Design review of the part built by this model. Coordinates are the model's own, in mm. Coordinates: 2 decimals unless noted, no trailing zeros. Loops run counter-clockwise (first coordinate to the right, second up) from the corner with the lowest first, then second, coordinate; pieces in that order, holes last. Notation, with made-up numbers: M -6,20.25 L 18,20.25 A31 ccw 18,48.25 Z; hole C 88,40 d9. An arc over 180 degrees is marked long. Answer as a JSON object with one key per item and string values. Group by question number.
1. To check wall thickness, follow probe 1 along Y at (x, z) = (1.25, 1); probe 2 along Y at (x, z) = (0.25, 0.35); probe 3 along X at (y, z) = (1, 0.5). State the ranges of each line that lie inside material, in increasing order.
2. Insertion check: pin 1 (1 mm diameter, centred on x = 1.5, z = 1.5, fed in from -Y); pin 2 (3 mm diameter, centred on x = 0, y = 0, fed in from +Z). Each pin has a flat end and moves straight along its axis. Give the tip position at first contact, or say it passes through.
3. Consider section B-B (z = 2.7). State the section outline as (x, y) points, then the cut area to 3 significant figures.
4. Consider section A-A (z = 1.35). State the section outline as (x, y) points.
5. Draft analysis for pull direction X (two halves, no side actions). For faces 1 (the conical face through (-3.14, 1.82, 2.87)), 2 (the flat face through (2, -2, 0)), 3 (the cylindrical face through (0, -2, 1)), state which applies: +X half, -X half, draft (parallel to the pull), parting line (faces both ways), or undercut.
from build123d import *

# Parameters (mm, degrees)
SKETCH1_R               = 2
BOSS_EXTRUDE1_DEPTH     = 3
SKETCH2_OUTSIDE_W       = 17.222
SKETCH2_OUTSIDE_H       = 18.304
SKETCH2_OUTSIDE_R       = 3.5
CUT_EXTRUDE1_DEPTH      = 3
CUT_EXTRUDE1_DRAFT      = -45
MIRROR1_COPY_1_SKETCH_W = 17.222
MIRROR1_COPY_1_SKETCH_H = 18.304
MIRROR1_COPY_1_SKETCH_R = 3.5
MIRROR1_COPY_1_DEPTH    = 3
MIRROR1_COPY_1_DRAFT    = -45


with BuildPart() as part:
    # Sketch1 → Boss-Extrude1 (new body)
    with BuildSketch(Plane.XY):
        Polygon((3.5, 2.020725942), (0, 4.041451884), (-3.5, 2.020725942), (-3.5, -2.020725942), (0, -4.041451884), (3.5, -2.020725942), align=None)
        Circle(SKETCH1_R, mode=Mode.SUBTRACT)
    extrude(amount=BOSS_EXTRUDE1_DEPTH)


with BuildPart() as cut_extrude1_tool:
    # Sketch2 outside → Cut-Extrude1 (with draft: the straight prism first)
    with BuildSketch(Plane.XY.offset(3)):
        Rectangle(SKETCH2_OUTSIDE_W, SKETCH2_OUTSIDE_H)
        Circle(SKETCH2_OUTSIDE_R, mode=Mode.SUBTRACT)
    extrude(amount=-CUT_EXTRUDE1_DEPTH)
    # Cut-Extrude1: the draft: its side faces are tilted about the plane it starts from
    cut_extrude1_sides = [cut_extrude1_tool.faces().sort_by_distance(p)[0] for p in [
        (0, -9.152, 1.5),
        (8.611, 0, 1.5),
        (0, 9.152, 1.5),
        (-8.611, 0, 1.5),
        (-3.5, 0, 1.5),
    ]]
    draft(cut_extrude1_sides, Plane.XY.offset(3), CUT_EXTRUDE1_DRAFT)


with BuildPart() as part_1:
    add(part.part)

    # Cut-Extrude1: cut by cut_extrude1_tool
    add(cut_extrude1_tool.part, mode=Mode.SUBTRACT)


with BuildPart() as mirror1_copy_1_tool:
    # Mirror1 copy 1 sketch → Mirror1 copy 1 (with draft: the straight prism first)
    with BuildSketch(Plane(origin=(0, 0, 0), x_dir=(1, 0, 0), z_dir=(0, 0, -1))):
        Rectangle(MIRROR1_COPY_1_SKETCH_W, MIRROR1_COPY_1_SKETCH_H)
        Circle(MIRROR1_COPY_1_SKETCH_R, mode=Mode.SUBTRACT)
    extrude(amount=-MIRROR1_COPY_1_DEPTH)
    # Mirror1 copy 1: the draft: its side faces are tilted about the plane it starts from
    mirror1_copy_1_sides = [mirror1_copy_1_tool.faces().sort_by_distance(p)[0] for p in [
        (0, -9.152, 1.5),
        (8.611, 0, 1.5),
        (0, 9.152, 1.5),
        (-8.611, 0, 1.5),
        (-3.5, 0, 1.5),
    ]]
    draft(mirror1_copy_1_sides, Plane(origin=(0, 0, 0), x_dir=(1, 0, 0), z_dir=(0, 0, -1)), MIRROR1_COPY_1_DRAFT)


with BuildPart() as part_2:
    add(part_1.part)

    # Mirror1 copy 1: cut by mirror1_copy_1_tool
    add(mirror1_copy_1_tool.part, mode=Mode.SUBTRACT)


solid = part_2.part
Findings below:
{
 "1": {"probe 1": "y = -3.32 to -1.56, 1.56 to 3.32", "probe 2": "y = -3.84 to -1.98, 1.98 to 3.84", "probe 3": "x = -3.5 to -1.73, 1.73 to 3.5"},
 "2": {"pin 1": "stops at y = -3.46", "pin 2": "passes through"},
 "3": {"outline": "M -3.5,-1.48 A3.8 ccw -3.03,-2.29 L -0.47,-3.77 A3.8 ccw 0.47,-3.77 L 3.03,-2.29 A3.8 ccw 3.5,-1.48 L 3.5,1.48 A3.8 ccw 3.03,2.29 L 0.47,3.77 A3.8 ccw -0.47,3.77 L -3.03,2.29 A3.8 ccw -3.5,1.48 Z; hole C 0,0 d4", "area": "29.2 mm^2"},
 "4": {"outline": "M -3.5,-2.02 L 0,-4.04 L 3.5,-2.02 L 3.5,2.02 L 0,4.04 L -3.5,2.02 Z; hole C 0,0 d4"},
 "5": {"face 1": "-X half", "face 2": "draft", "face 3": "undercut"}
}
